Geometry: see drawing. Coordinates: mm, zero at the bounding-box minimum. A direction names the side the tool comes from. Coordinates: 2 decimals unless noted, no trailing zeros. Order: outer loops, then holes, each group sorted by start corner. A loop starts at its lowest first (then second) coordinate and runs counter-clockwise, first axis right, second up. Notation, with made-up numbers: (49.25, -22.75) -> (96.25, -22.75) arc R11 cw to (96.25, -8.75) -> close; hole circle Ø3 at (29, 51). An arc over 180 degrees is marked (long way). Use one line per item in the form item = value.
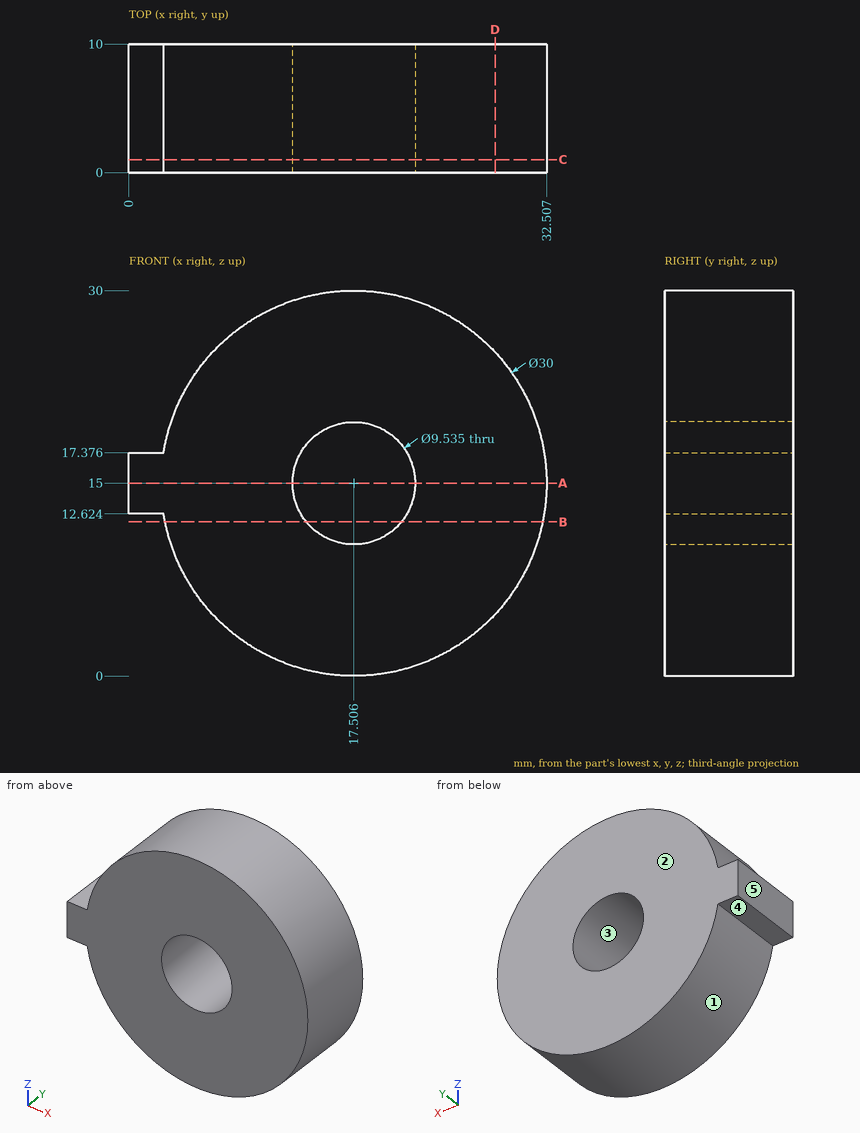
1) Section C-C, the plane y = 1. Output: boundary loops of the cut face in (x, z) (1 decimal).
Results found:
outline = (0, 12.6) -> (2.7, 12.6) arc R15 ccw (long way) to (2.7, 17.4) -> (0, 17.4) -> close; hole circle Ø9.5 at (17.5, 15)
2) Section A-A, the plane z = 15. Output: boundary loops of the cut face in (x, y), and give its area (3 significant figures).
Results found:
outline = (0, 0) -> (12.74, 0) -> (12.74, 10) -> (0, 10) -> close; (22.27, 0) -> (32.51, 0) -> (32.51, 10) -> (22.27, 10) -> close
area = 230 mm2
3) Pull-direction query (X, two-part tool) for the marked faces 1, 2 and 3; classes: released by +X, released by -X, zero draft, split by the parting line, or undercut.
Results found:
face_1 = split by the parting line
face_2 = zero draft
face_3 = undercut
4) Access query for the marked faces 4 and 5. Directions: +Z, -Z, +X, -X, +Y, -Y. A direction counts if a zero-diameter tool reaches every point of the face in a straight line with its end or side. Return the directions, or none.
Results found:
face_4 = -Z, -X, +Y, -Y
face_5 = +Z, -Z, -X, +Y, -Y
5) Section B-B, the plane z = 12. Output: boundary loops of the cut face in (x, y), and give its area (3 significant figures).
Results found:
outline = (2.81, 0) -> (13.8, 0) -> (13.8, 10) -> (2.81, 10) -> close; (21.21, 0) -> (32.2, 0) -> (32.2, 10) -> (21.21, 10) -> close
area = 220 mm2
6) Section D-D, the plane x = 28.5. Output: boundary loops of the cut face in (y, z) (1 decimal).
Results found:
outline = (0, 4.8) -> (10, 4.8) -> (10, 25.2) -> (0, 25.2) -> close
7) Material intervals for probe 1 along Z at (x, y) = (1, 3.75); probe 2 along Z at (x, y) = (21.5, 6.5) (1 decimal); probe 3 along X at (y, z) = (4.25, 12.5) (1 decimal), sorted ascending. Write a range as from..to.
Results found:
probe_1 = 12.62..17.38
probe_2 = 0.5..12.4, 17.6..29.5
probe_3 = 2.7..13.4, 21.6..32.3
8) Contact query for flat-ended pins moving along their axis: P1, Ø5, axis at y = 8, z = 10, coming from the -X side; P2, Ø2, axis at y = 4.5, z = 11, coming from the +X side; P3, Ø1, axis at y = 3, z = 22, coming from the -X side. Output: stop coordinate, or through.
Results found:
P1 = 2.72
P2 = 32.2
P3 = 3.99
